Input: part model. Units: mm. Frame: model coordinates. A direction names the side the tool comes from. Coordinates: 2 decimals unless noted, no trailing zeros. Order: outer loops, then holes, each group sorted by start corner. A loop starts at its lowest first (then second) coordinate and runs counter-clockwise, first axis right, second up. Notation, with made-up numbers: (-5, 21.5) -> (44, 21.5) arc R26 ccw to (44, 50.5) -> close; hole circle Ø1 at (-34.75, 86.25). An arc over 180 degrees is marked (long way). One line per item, written item: value. Start each with the question number.
from build123d import *

# Parameters (mm, degrees)
F0_W     = 101.6
F0_H     = 165.1
F0_R     = 15.875
F1_DEPTH = 76.2
F2_W     = 139.7
F2_H     = 158.75
F3_DEPTH = 101.601
F4_R     = 12.7
F5_DEPTH = 73.025
F7_DEPTH = 88.9
F8_R     = 4.7625


with BuildPart() as f1:
    # F0 (on Right) → F1 (new body, symmetric)
    with BuildSketch(Plane.YZ):
        Rectangle(F0_W, F0_H)
        with Locations((-25.4, -57.15)):
            Circle(F0_R, mode=Mode.SUBTRACT)
        with Locations((-25.4, 0)):
            Circle(F0_R, mode=Mode.SUBTRACT)
        with Locations((25.4, -28.575)):
            Circle(F0_R, mode=Mode.SUBTRACT)
        with Locations((-25.4, 57.15)):
            Circle(F0_R, mode=Mode.SUBTRACT)
        with Locations((25.4, 28.575)):
            Circle(F0_R, mode=Mode.SUBTRACT)
        with Locations((-25.4, 57.15)):
            Circle(F0_R)
        with Locations((25.4, 28.575)):
            Circle(F0_R)
        with Locations((-25.4, 0)):
            Circle(F0_R)
        with Locations((25.4, -28.575)):
            Circle(F0_R)
        with Locations((-25.4, -57.15)):
            Circle(F0_R)
    extrude(amount=F1_DEPTH, both=True)

    # F2 (on face) → F3 (cut, through all)
    with BuildSketch(Plane.XZ.offset(50.8)):
        with Locations((0, 3.175)):
            Rectangle(F2_W, F2_H)
    extrude(amount=-F3_DEPTH, mode=Mode.SUBTRACT)

    # F4 (on Right) → F5 (join, symmetric)
    with BuildSketch(Plane.YZ):
        with Locations((-15.875, 47.625)):
            Circle(F4_R)
        with Locations((28.575, 23.8125)):
            Circle(F4_R)
        with Locations((-15.875, 0)):
            Circle(F4_R)
        with Locations((28.575, -23.8125)):
            Circle(F4_R)
        with Locations((-15.875, -47.625)):
            Circle(F4_R)
    extrude(amount=F5_DEPTH, both=True)

    # F6 (on Right) → F7 (join, symmetric)
    with BuildSketch(Plane.YZ):
        Polygon((-50.8, 82.55), (50.8, 82.55), (69.85, 82.55), (69.85, 88.519), (-88.9, 88.519), (-88.9, 82.55), align=None)
    extrude(amount=F7_DEPTH, both=True)

    # F10: sweep along a path in F9
    with BuildLine(Plane.XZ) as f10_path:
        Line((-60.325, 88.519), (-60.325, 107.569))
        ThreePointArc((-60.325, 107.569), (-54.7453841816, 121.0393841816), (-41.275, 126.619))
        Line((-41.275, 126.619), (41.275, 126.619))
        ThreePointArc((41.275, 126.619), (54.7453841816, 121.0393841816), (60.325, 107.569))
        Line((60.325, 107.569), (60.325, 88.519))
    # F8 (on face) → F10 (sweep)
    with BuildSketch(Plane.XY.offset(88.519)):
        with Locations((-60.325, 0)):
            Circle(F8_R)
    sweep(path=f10_path.line)


solid = f1.part
1) Pin query (flat end, axial travel): pin 1 Ø5 at (y, z) = (41.5, -54) entering from -X; pin 2 Ø12 at (y, z) = (22.5, -27.5) entering from +X; pin 3 Ø8 at (x, z) = (-36, -10.5) entering from -Y. Return the tip coordinate at first contact, or that it passes through.
2) Ray query, line 1 along Z through (x, y) = (-37.5, -46.5); line 2 along X through (y, z) = (-44, -35); line 3 along Z through (x, y) = (-29.5, 35.5). Return the intervals inside material, ascending. Write a range as from..to.
3) Section query C-C, the plane y = 30. Return the cut outline in (x, z), plus the area to 3 significant figures.
4) Section query A-A, the plane y = 0. State how many separate pieces and enclosed holes the cut face has, plus the area to 3 significant figures.
5) Section query B-B, the plane z = 0. Return the cut outline in (x, y) (3 decimals), plus the area to 3 significant figures.
6) Mould query, pull axis Z, two halves, no side actions, for faces 1 (the flat face through (0, -50.8, -80)), 2 (the cylindrical face through (0.978, -18.628, -60.023)), 3 (the flat face through (1, -1, -82.55)). Classes: +Z half, -Z half, draft (parallel to the pull), parting line (faces both ways), or undercut.
7) Access query for faces 4 (the cylindrical face through (65.083, 0.209, 97.911)), 5 (the flat face through (0, 50.8, -80)), 6 (the flat face through (-1, -1, -76.2)), 7 (the flat face through (76.2, -1, 1)). Directions: +Z, -Z, +X, -X, +Y, -Y. A direction counts if a zero-diameter tool reaches every point of the face in a straight line with its end or side. Return the directions, or none.
Entries:
1. pin 1: stops at x = -76.2
1. pin 2: stops at x = 76.2
1. pin 3: stops at y = -26.79
2. line 1: z = -82.55..-76.2, 82.55..88.52
2. line 2: x = -76.2..-69.85, 69.85..76.2
2. line 3: z = -82.55..-76.2, -34.46..-13.17, 13.17..34.46, 82.55..88.52
3. outline: (-88.9, 82.55) -> (-76.2, 82.55) -> (-76.2, -82.55) -> (76.2, -82.55) -> (76.2, 82.55) -> (88.9, 82.55) -> (88.9, 88.52) -> (-88.9, 88.52) -> close; hole (-69.85, -76.2) -> (69.85, -76.2) -> (69.85, -36.43) -> (-69.85, -36.43) -> close; hole (-69.85, -11.19) -> (69.85, -11.19) -> (69.85, 11.19) -> (-69.85, 11.19) -> close; hole (-69.85, 36.43) -> (69.85, 36.43) -> (69.85, 82.55) -> (-69.85, 82.55) -> close
3. area: 11,100 mm2
4. separate pieces: 1
4. enclosed holes: 2
4. area: 5,760 mm2
5. outline: (-76.2, -50.8) -> (-69.85, -50.8) -> (-69.85, -28.575) -> (69.85, -28.575) -> (69.85, -50.8) -> (76.2, -50.8) -> (76.2, 50.8) -> (69.85, 50.8) -> (69.85, -3.175) -> (-69.85, -3.175) -> (-69.85, 50.8) -> (-76.2, 50.8) -> close
5. area: 4,840 mm2
6. face 1: draft
6. face 2: undercut
6. face 3: -Z half
7. face 4: none
7. face 5: -Z, +X, -X, +Y
7. face 6: +Y, -Y
7. face 7: -Z, +X, +Y, -Y
